Geometry: final body of the model. Coordinates: model frame, mm. A direction names the side the tool comes from. Round coordinates to 2 decimals unless told otherwise and drop trailing zeros. Loops run counter-clockwise (first coordinate to the right, second up) from the corner with the lowest first, then second, coordinate; pieces in that order, holes last. Notation, with made-up numbers: (25, 33) - (77, 33) arc R11 cw to (77, 43) - close; hole circle Ø10 at (20.5, 87.25). An arc over 180 degrees is marked (long way). Use CSV: the item, a comma, the result in double quotes.
from build123d import *

# Parameters (mm, degrees)
F0_R      = 73.9775
F1_DEPTH  = 21.59
F3_DEPTH  = 21.591
F4_R      = 38.1
F5_DEPTH  = 21.59
F6_R      = 16.51
F7_DEPTH  = 25.4
F9_D      = 19.05
F10_W     = 6.35
F10_H     = 6.35
F11_DEPTH = 25.4


with BuildPart() as f1:
    # F0 (on Top) → F1 (new body)
    with BuildSketch(Plane.XY):
        Circle(F0_R)
    extrude(amount=F1_DEPTH)

    # F2 (on face) → F3 (cut, through all)
    with BuildSketch(Plane.XY.offset(21.59)):
        with BuildLine():
            ThreePointArc((-45.649791, 32.228419), (-42.736956, 36.001764), (-39.513127, 39.513127))
            ThreePointArc((-39.513127, 39.513127), (-36.001764, 42.736956), (-32.228419, 45.649791))
            ThreePointArc((-32.228419, 45.649791), (-46.248319, 46.248319), (-45.649791, 32.228419))
        make_face()
        with BuildLine():
            Line((-39.513127, 39.513127), (-32.777935, 32.777935))
            ThreePointArc((-32.777935, 32.777935), (-30.713174, 35.868067), (-29.988127, 39.513127))
            ThreePointArc((-29.988127, 39.513127), (-30.565712, 42.77953), (-32.228419, 45.649791))
            ThreePointArc((-32.228419, 45.649791), (-36.001764, 42.736956), (-39.513127, 39.513127))
        make_face()
        with BuildLine():
            ThreePointArc((-45.649791, 32.228419), (-39.106862, 29.996795), (-32.777935, 32.777935))
            Line((-32.777935, 32.777935), (-39.513127, 39.513127))
            ThreePointArc((-39.513127, 39.513127), (-42.736956, 36.001764), (-45.649791, 32.228419))
        make_face()
        with BuildLine():
            ThreePointArc((-9.490344, 55.06821), (-4.7625, 55.676683), (0, 55.88))
            ThreePointArc((0, 55.88), (4.7625, 55.676683), (9.490344, 55.06821))
            ThreePointArc((9.490344, 55.06821), (9.516332, 55.473735), (9.525, 55.88))
            ThreePointArc((9.525, 55.88), (-0.406265, 65.396332), (-9.490344, 55.06821))
        make_face()
        with BuildLine():
            Line((0, 55.88), (0, 46.355))
            ThreePointArc((0, 46.355), (6.44179, 48.863665), (9.490344, 55.06821))
            ThreePointArc((9.490344, 55.06821), (4.7625, 55.676683), (0, 55.88))
        make_face()
        with BuildLine():
            ThreePointArc((-9.490344, 55.06821), (-6.44179, 48.863665), (0, 46.355))
            Line((0, 46.355), (0, 55.88))
            ThreePointArc((0, 55.88), (-4.7625, 55.676683), (-9.490344, 55.06821))
        make_face()
        with BuildLine():
            ThreePointArc((32.777935, 32.777935), (39.106862, 29.996795), (45.649791, 32.228419))
            ThreePointArc((45.649791, 32.228419), (42.736956, 36.001764), (39.513127, 39.513127))
            Line((39.513127, 39.513127), (32.777935, 32.777935))
        make_face()
        with BuildLine():
            Line((32.777935, 32.777935), (39.513127, 39.513127))
            ThreePointArc((39.513127, 39.513127), (36.001764, 42.736956), (32.228419, 45.649791))
            ThreePointArc((32.228419, 45.649791), (29.996795, 39.106862), (32.777935, 32.777935))
        make_face()
        with BuildLine():
            ThreePointArc((39.513127, 39.513127), (42.736956, 36.001764), (45.649791, 32.228419))
            ThreePointArc((45.649791, 32.228419), (48.149601, 35.496045), (49.038127, 39.513127))
            ThreePointArc((49.038127, 39.513127), (42.77953, 48.460542), (32.228419, 45.649791))
            ThreePointArc((32.228419, 45.649791), (36.001764, 42.736956), (39.513127, 39.513127))
        make_face()
        with BuildLine():
            ThreePointArc((55.06821, -9.490344), (55.676683, -4.7625), (55.88, 0))
            Line((55.88, 0), (46.355, 0))
            ThreePointArc((46.355, 0), (48.863665, -6.44179), (55.06821, -9.490344))
        make_face()
        with BuildLine():
            ThreePointArc((55.06821, 9.490344), (55.676683, 4.7625), (55.88, 0))
            ThreePointArc((55.88, 0), (55.676683, -4.7625), (55.06821, -9.490344))
            ThreePointArc((55.06821, -9.490344), (62.32179, -7.016335), (65.405, 0))
            ThreePointArc((65.405, 0), (62.32179, 7.016335), (55.06821, 9.490344))
        make_face()
        with BuildLine():
            Line((46.355, 0), (55.88, 0))
            ThreePointArc((55.88, 0), (55.676683, 4.7625), (55.06821, 9.490344))
            ThreePointArc((55.06821, 9.490344), (48.863665, 6.44179), (46.355, 0))
        make_face()
        with BuildLine():
            ThreePointArc((32.228419, -45.649791), (36.001764, -42.736956), (39.513127, -39.513127))
            Line((39.513127, -39.513127), (32.777935, -32.777935))
            ThreePointArc((32.777935, -32.777935), (29.996795, -39.106862), (32.228419, -45.649791))
        make_face()
        with BuildLine():
            ThreePointArc((39.513127, -39.513127), (42.736956, -36.001764), (45.649791, -32.228419))
            ThreePointArc((45.649791, -32.228419), (39.106862, -29.996795), (32.777935, -32.777935))
            Line((32.777935, -32.777935), (39.513127, -39.513127))
        make_face()
        with BuildLine():
            ThreePointArc((49.038127, -39.513127), (48.149601, -35.496045), (45.649791, -32.228419))
            ThreePointArc((45.649791, -32.228419), (42.736956, -36.001764), (39.513127, -39.513127))
            ThreePointArc((39.513127, -39.513127), (36.001764, -42.736956), (32.228419, -45.649791))
            ThreePointArc((32.228419, -45.649791), (42.77953, -48.460542), (49.038127, -39.513127))
        make_face()
        with BuildLine():
            ThreePointArc((9.490344, -55.06821), (6.44179, -48.863665), (0, -46.355))
            Line((0, -46.355), (0, -55.88))
            ThreePointArc((0, -55.88), (4.7625, -55.676683), (9.490344, -55.06821))
        make_face()
        with BuildLine():
            Line((0, -55.88), (0, -46.355))
            ThreePointArc((0, -46.355), (-6.44179, -48.863665), (-9.490344, -55.06821))
            ThreePointArc((-9.490344, -55.06821), (-4.7625, -55.676683), (0, -55.88))
        make_face()
        with BuildLine():
            ThreePointArc((9.490344, -55.06821), (4.7625, -55.676683), (0, -55.88))
            ThreePointArc((0, -55.88), (-4.7625, -55.676683), (-9.490344, -55.06821))
            ThreePointArc((-9.490344, -55.06821), (-0.406265, -65.396332), (9.525, -55.88))
            ThreePointArc((9.525, -55.88), (9.516332, -55.473735), (9.490344, -55.06821))
        make_face()
        with BuildLine():
            ThreePointArc((-32.228419, -45.649791), (-36.001764, -42.736956), (-39.513127, -39.513127))
            ThreePointArc((-39.513127, -39.513127), (-42.736956, -36.001764), (-45.649791, -32.228419))
            ThreePointArc((-45.649791, -32.228419), (-46.248319, -46.248319), (-32.228419, -45.649791))
        make_face()
        with BuildLine():
            ThreePointArc((-29.988127, -39.513127), (-30.713174, -35.868067), (-32.777935, -32.777935))
            Line((-32.777935, -32.777935), (-39.513127, -39.513127))
            ThreePointArc((-39.513127, -39.513127), (-36.001764, -42.736956), (-32.228419, -45.649791))
            ThreePointArc((-32.228419, -45.649791), (-30.565712, -42.77953), (-29.988127, -39.513127))
        make_face()
        with BuildLine():
            Line((-39.513127, -39.513127), (-32.777935, -32.777935))
            ThreePointArc((-32.777935, -32.777935), (-39.106862, -29.996795), (-45.649791, -32.228419))
            ThreePointArc((-45.649791, -32.228419), (-42.736956, -36.001764), (-39.513127, -39.513127))
        make_face()
        with BuildLine():
            ThreePointArc((-55.06821, -9.490344), (-55.676683, -4.7625), (-55.88, 0))
            ThreePointArc((-55.88, 0), (-55.676683, 4.7625), (-55.06821, 9.490344))
            ThreePointArc((-55.06821, 9.490344), (-65.405, 0), (-55.06821, -9.490344))
        make_face()
        with BuildLine():
            Line((-55.88, 0), (-46.355, 0))
            ThreePointArc((-46.355, 0), (-48.863665, 6.44179), (-55.06821, 9.490344))
            ThreePointArc((-55.06821, 9.490344), (-55.676683, 4.7625), (-55.88, 0))
        make_face()
        with BuildLine():
            ThreePointArc((-55.06821, -9.490344), (-48.863665, -6.44179), (-46.355, 0))
            Line((-46.355, 0), (-55.88, 0))
            ThreePointArc((-55.88, 0), (-55.676683, -4.7625), (-55.06821, -9.490344))
        make_face()
    extrude(amount=-F3_DEPTH, mode=Mode.SUBTRACT)

    # F4 (on face) → F5 (join)
    with BuildSketch(Plane.XY.offset(21.59)):
        Circle(F4_R)
    extrude(amount=F5_DEPTH)

    # F6 (on face) → F7 (join)
    with BuildSketch(Plane.XY.offset(43.18)):
        Circle(F6_R)
    extrude(amount=F7_DEPTH)

    # F9 (through all)
    with Locations(Plane.XY.offset(68.58)):
        with Locations((0, 0)):
            Hole(F9_D / 2)

    # F10 (on face) → F11 (cut)
    with BuildSketch(Plane.XY.offset(68.58)):
        with Locations((0, -9.525)):
            Rectangle(F10_W, F10_H)
    extrude(amount=-F11_DEPTH, mode=Mode.SUBTRACT)


solid = f1.part
Item 1: Reachability of faces 1 (the flat face through (3.175, -11, 56)), 2 (the flat face through (7, -7, 68.58)) from +Z, -Z, +X, -X, +Y, -Y: full face, straight path, thin tool, end or side. Return the list, or none.
Final values:
face 1,"+Z"
face 2,"+Z, +X, -X, +Y, -Y"
Item 2: Section B-B on x = -51.5. Return the cut outline in (y, z), plus the area to 3 significant figures.
Final values:
outline,"(-53.11, 0) - (-8.46, 0) - (-8.46, 21.59) - (-53.11, 21.59) - close; (8.46, 0) - (53.11, 0) - (53.11, 21.59) - (8.46, 21.59) - close"
area,"1,930 mm²"
Item 3: Section A-A on z = 6. Give the number of separate pieces and of enclosed holes in the cut face, plus the area to 3 significant figures.
Final values:
separate pieces,"1"
enclosed holes,"9"
area,"14,600 mm²"
Item 4: Mould query, pull axis X, two halves, no side actions, for faces 3 (the flat face through (0, -11, 43.18)), 4 (the flat face through (0, -12.7, 56)), 5 (the cylindrical face through (15.748, 4.959, 55.702)), 6 (the flat face through (15, 1, 0)). Classes: released by +X, released by -X, zero draft, split by the parting line, or undercut.
Final values:
face 3,"undercut"
face 4,"undercut"
face 5,"split by the parting line"
face 6,"zero draft"
Item 5: Pin query (flat end, axial travel): P1, Ø10, axis at x = 53, z = 20.5, coming from the +Y side; P2, Ø2, axis at x = 9.5, z = 53, coming from the +Y side; P3, Ø3, axis at y = -19.5, z = 18, coming from the +X side; P4, Ø22, axis at x = 0, y = 0, coming from the +Z side. Return the tip coordinate at first contact, or that it passes through.
Final values:
P1,"stops at y = 56.29"
P2,"stops at y = 14.15"
P3,"stops at x = 71.75"
P4,"stops at z = 68.58"
Item 6: Material intervals for line 1 (Y direction, x = -5.5, z = 12); line 2 (Y direction, x = -3.5, z = 15), sorted ascending.
Final values:
line 1,"y = -73.77 to -63.66, -48.1 to -7.78, 7.78 to 48.1, 63.66 to 73.77"
line 2,"y = -73.89 to -64.74, -47.02 to -8.86, 8.86 to 47.02, 64.74 to 73.89"
Item 7: Section D-D on z = 61.5. Return the cut outline in (x, y) (3 decimals).
Final values:
outline,"circle Ø33.02 at (0, 0); hole (-3.175, -12.7) - (3.175, -12.7) - (3.175, -8.98) arc R9.525 ccw (long way) to (-3.175, -8.98) - close"
Item 8: Section C-C on y = 59. Return the cut outline in (x, z), plus the area to 3 significant figures.
Final values:
outline,"(-44.63, 0) - (-9, 0) - (-9, 21.59) - (-44.63, 21.59) - close; (9, 0) - (44.63, 0) - (44.63, 21.59) - (9, 21.59) - close"
area,"1,540 mm²"
